Build history of the part. All positions in model axes, mm. A direction names the side the tool comes from. Give positions to 0.01 mm unless a question says otherwise; leave off trailing zeros. Loops run counter-clockwise (first coordinate to the right, second up) from the corner with the lowest first, then second, coordinate; pieces in that order, holes last. Notation, with made-up numbers: (-19.5, 18) -> (30.5, 18) arc R25 cw to (30.5, 56) -> close; hole circle Ø10 at (68.5, 7.25). An arc over 180 degrees is marked (long way). Answer as a JSON object with one key per item and string values. Group by question number.
Q1. Two-plate mould, pull along X, no slides. Class faces 1 (the flat face through (22.08, 23.81, 52.32)), 2 (the flat face through (-0.1, -19.05, -7.4)), 3 (the cylindrical face through (-0.849, 27.361, -94.976)), 4 (the cylindrical face through (-1.86, -180.32, 32.36)): pulls with the +X half, pulls with the -X half, needs draft (parallel to the pull), parting line crosses it, or undercut.
Q2. Band-saw the part on C-C, the plane z = -60.5. Write the cut outline in (x, y).
Q3. Wall check: probe 1 along Z at (x, y) = (-1.5, -213); probe 2 along Y at (x, z) = (-24.5, -5.5); probe 3 along Y at (x, z) = (16.5, 35). Give the ranges that are in metal, low to high. Write a range as from..to.
Q4. Tool access for faces 5 (the flat face through (-38.595, 24, -6)), 6 (the cylindrical face through (15.56, -13.85, 42.6)), 7 (the flat face through (0, -114.986, -56)), 8 (the cylindrical face through (10.31, 77.045, 10.206)), 9 (the flat face through (-1, -4, -19.311)): list every direction of +Z, -Z, +X, -X, +Y, -Y with a clear straight run to the whole face (end or side of a thin tool).
Q5. Band-saw the part on D-D, the plane y = -204. Write the cut outline in (x, z) (1 decimal), plus the area to 3 significant figures.
Q6. Drop flat-ended pins along their axis: pin 1 (11.5 mm diameter, centred on y = 79.98, z = 17.82, fed in from +X); pin 2 (9.5 mm diameter, centred on x = 7, y = -6, fed in from -Z); pin 3 (22.5 mm diameter, centred on x = 17.5, z = -52.5, fed in from -Y); pin 4 (12 mm diameter, centred on x = 25, y = -194.5, fed in from +Z). Give the stop position or say it passes through.
Q7. Band-saw the part on B-B, the plane y = 40. Write the cut outline in (x, z), plus the area to 3 significant figures.
from build123d import *

# Parameters (mm, degrees)
F0_R      = 28.9450820598
F0_R_2    = 31.75
F0_R_3    = 25.3342985941
F0_R_4    = 14.2875
F1_DEPTH  = 55.499
F2_DEPTH  = 114.9858
F3_DEPTH  = 365.76
F4_DEPTH  = 8.7884
F5_DEPTH  = 19.05
F6_R      = 12.9921
F7_DEPTH  = 38.481
F6_R_2    = 19.0658392813
F8_DEPTH  = 5.07789
F9_R      = 6.4897
F10_DEPTH = 25.4
F11_DEPTH = 25.4


with BuildPart() as f1:
    # F0 (on Front) → F1 (new body)
    with BuildSketch(Plane.XZ):
        with BuildLine():
            ThreePointArc((-34.3382090481, 48.0584091192), (-37.4227739234, 45.7396722427), (-38.5953, 42.0632250756))
            Line((-38.5953, 42.0632250756), (-38.5953, -19.3111319095))
            Line((-38.5953, -19.3111319095), (38.5953, -19.3111319095))
            Line((38.5953, -19.3111319095), (38.5953, 42.0582217318))
            ThreePointArc((38.5953, 42.0582217318), (37.4208481647, 45.7373794064), (34.331929545, 48.0555942517))
            Line((34.331929545, 48.0555942517), (9.4760187225, 56.7035609601))
            Line((9.4760187225, 56.7035609601), (-9.5739812775, 56.7035609601))
            Line((-9.5739812775, 56.7035609601), (-34.3382090481, 48.0584091192))
        make_face()
        with Locations((0, 18.1938651949)):
            Circle(F0_R, mode=Mode.SUBTRACT)
        with BuildLine():
            Line((38.5953, -19.3111319095), (-38.5953, -19.3111319095))
            Line((-38.5953, -19.3111319095), (-38.5953, -56.3899390399))
            ThreePointArc((-38.5953, -56.3899390399), (0, -94.9852390399), (38.5953, -56.3899390399))
            Line((38.5953, -56.3899390399), (38.5953, -19.3111319095))
        make_face()
        with Locations((0, -56.3899390399)):
            Circle(F0_R_2, mode=Mode.SUBTRACT)
        with Locations((0, -56.3899390399)):
            Circle(F0_R_2)
        with Locations((0, 18.1938651949)):
            Circle(F0_R)
        with Locations((0, 18.1938651949)):
            Circle(F0_R_3, mode=Mode.SUBTRACT)
        with Locations((0, 18.1938651949)):
            Circle(F0_R_3)
        with Locations((0, 18.1938651949)):
            Circle(F0_R_4, mode=Mode.SUBTRACT)
        with Locations((0, 18.1938651949)):
            Circle(F0_R_4)
    extrude(amount=-F1_DEPTH)

    # F0 (on Front) → F2 (join)
    with BuildSketch(Plane.XZ):
        with Locations((0, -56.3899390399)):
            Circle(F0_R_2)
    extrude(amount=F2_DEPTH)

    # F0 (on Front) → F3 (join)
    with BuildSketch(Plane.XZ):
        with Locations((0, 18.1938651949)):
            Circle(F0_R_3)
        with Locations((0, 18.1938651949)):
            Circle(F0_R_4, mode=Mode.SUBTRACT)
    extrude(amount=F3_DEPTH)

    # F0 (on Front) → F4 (join)
    with BuildSketch(Plane.XZ):
        with BuildLine():
            ThreePointArc((-34.3382090481, 48.0584091192), (-37.4227739234, 45.7396722427), (-38.5953, 42.0632250756))
            Line((-38.5953, 42.0632250756), (-38.5953, -19.3111319095))
            Line((-38.5953, -19.3111319095), (38.5953, -19.3111319095))
            Line((38.5953, -19.3111319095), (38.5953, 42.0582217318))
            ThreePointArc((38.5953, 42.0582217318), (37.4208481647, 45.7373794064), (34.331929545, 48.0555942517))
            Line((34.331929545, 48.0555942517), (9.4760187225, 56.7035609601))
            Line((9.4760187225, 56.7035609601), (-9.5739812775, 56.7035609601))
            Line((-9.5739812775, 56.7035609601), (-34.3382090481, 48.0584091192))
        make_face()
        with Locations((0, 18.1938651949)):
            Circle(F0_R, mode=Mode.SUBTRACT)
    extrude(amount=F4_DEPTH)

    # F0 (on Front) → F5 (join)
    with BuildSketch(Plane.XZ):
        with Locations((0, 18.1938651949)):
            Circle(F0_R)
        with Locations((0, 18.1938651949)):
            Circle(F0_R_3, mode=Mode.SUBTRACT)
    extrude(amount=F5_DEPTH)

    # F6 (on face) → F7 (join)
    with BuildSketch(Plane(origin=(0, 55.499, 0), x_dir=(-1, 0, 0), z_dir=(0, 1, 0))):
        with Locations((0, 18.111359328)):
            Circle(F6_R)
    extrude(amount=F7_DEPTH)

    # F6 (on face) → F8 (join)
    with BuildSketch(Plane(origin=(0, 55.499, 0), x_dir=(-1, 0, 0), z_dir=(0, 1, 0))):
        with Locations((0, 18.111359328)):
            Circle(F6_R_2)
        with Locations((0, 18.111359328)):
            Circle(F6_R, mode=Mode.SUBTRACT)
    extrude(amount=F8_DEPTH)

    # F9 (on Right) → F10 (cut)
    with BuildSketch(Plane.YZ):
        with Locations((79.9846, 17.8194735199)):
            Circle(F9_R)
    extrude(amount=-F10_DEPTH, mode=Mode.SUBTRACT)

    # F9 (on Right) → F11 (cut, symmetric)
    with BuildSketch(Plane.YZ):
        with Locations((79.9846, 17.8194735199)):
            Circle(F9_R)
    extrude(amount=F11_DEPTH, both=True, mode=Mode.SUBTRACT)


solid = f1.part
Worked answers:
{
 "1": {"face 1": "pulls with the +X half", "face 2": "needs draft", "face 3": "parting line crosses it", "face 4": "undercut"},
 "2": {"outline": "(-38.38, 0) -> (-31.48, 0) -> (-31.48, -114.99) -> (31.48, -114.99) -> (31.48, 0) -> (38.38, 0) -> (38.38, 55.5) -> (-38.38, 55.5) -> close"},
 "3": {"probe 1": "-7.1..3.99, 32.4..43.48", "probe 2": "-8.79..55.5", "probe 3": "-365.76..55.5"},
 "4": {"face 5": "+Z, -Z, -X, +Y, -Y", "face 6": "-Y", "face 7": "-Z, +X, -X, -Y", "face 8": "+Y", "face 9": "+X, -X, -Y"},
 "5": {"outline": "circle Ø50.7 at (0, 18.2); hole circle Ø28.6 at (0, 18.2)", "area": "1,380 mm2"},
 "6": {"pin 1": "through", "pin 2": "z = -88.06", "pin 3": "y = -114.99", "pin 4": "z = 34.95"},
 "7": {"outline": "(-38.6, -56.39) arc R38.6 ccw to (38.6, -56.39) -> (38.6, 42.06) arc R6.35 ccw to (34.33, 48.06) -> (9.48, 56.7) -> (-9.57, 56.7) -> (-34.34, 48.06) arc R6.35 ccw to (-38.6, 42.06) -> close", "area": "10,800 mm2"}
}
